```python
from build123d import *

# Parameters (mm, degrees)
SKETCH1_R           = 2
SKETCH1_R_2         = 1.5
BOSS_EXTRUDE1_DEPTH = 3.175


with BuildPart() as part:
    # Sketch1 → Boss-Extrude1 (new body)
    with BuildSketch(Plane.XY):
        with BuildLine():
            Line((165, 154), (165, 99))
            Line((165, 99), (151, 85))
            Line((151, 85), (151, -85))
            Line((151, -85), (165, -99))
            Line((165, -99), (165, -154))
            ThreePointArc((165, -154), (161.778174593, -161.778174593), (154, -165))
            Line((154, -165), (99, -165))
            Line((99, -165), (85, -151))
            Line((85, -151), (-85, -151))
            Line((-85, -151), (-99, -165))
            Line((-99, -165), (-154, -165))
            ThreePointArc((-154, -165), (-161.778174593, -161.778174593), (-165, -154))
            Line((-165, -154), (-165, -99))
            Line((-165, -99), (-151, -85))
            Line((-151, -85), (-151, 85))
            Line((-151, 85), (-165, 99))
            Line((-165, 99), (-165, 154))
            ThreePointArc((-165, 154), (-161.778174593, 161.778174593), (-154, 165))
            Line((-154, 165), (-64, 165))
            Line((-64, 165), (-60, 169))
            Line((-60, 169), (60, 169))
            Line((60, 169), (64, 165))
            Line((64, 165), (154, 165))
            ThreePointArc((154, 165), (161.778174593, 161.778174593), (165, 154))
        make_face()
        with Locations((-14.5, -0.5)):
            Circle(SKETCH1_R, mode=Mode.SUBTRACT)
        with Locations((-93, 64)):
            Circle(SKETCH1_R, mode=Mode.SUBTRACT)
        with Locations((-93, 39)):
            Circle(SKETCH1_R, mode=Mode.SUBTRACT)
        with Locations((-57, 39)):
            Circle(SKETCH1_R, mode=Mode.SUBTRACT)
        with Locations((-57, 64)):
            Circle(SKETCH1_R, mode=Mode.SUBTRACT)
        with Locations((57, 39)):
            Circle(SKETCH1_R, mode=Mode.SUBTRACT)
        with Locations((57, 64)):
            Circle(SKETCH1_R, mode=Mode.SUBTRACT)
        with Locations((93, 39)):
            Circle(SKETCH1_R, mode=Mode.SUBTRACT)
        with Locations((93, 64)):
            Circle(SKETCH1_R, mode=Mode.SUBTRACT)
        with Locations((57, -64)):
            Circle(SKETCH1_R, mode=Mode.SUBTRACT)
        with Locations((57, -39)):
            Circle(SKETCH1_R, mode=Mode.SUBTRACT)
        with Locations((93, -39)):
            Circle(SKETCH1_R, mode=Mode.SUBTRACT)
        with Locations((93, -64)):
            Circle(SKETCH1_R, mode=Mode.SUBTRACT)
        with Locations((-93, -64)):
            Circle(SKETCH1_R, mode=Mode.SUBTRACT)
        with Locations((-57, -64)):
            Circle(SKETCH1_R, mode=Mode.SUBTRACT)
        with Locations((-57, -39)):
            Circle(SKETCH1_R, mode=Mode.SUBTRACT)
        with Locations((-93, -39)):
            Circle(SKETCH1_R, mode=Mode.SUBTRACT)
        with Locations((-20.5, -26.5)):
            Circle(SKETCH1_R, mode=Mode.SUBTRACT)
        with Locations((-161.5, 154)):
            Circle(SKETCH1_R_2, mode=Mode.SUBTRACT)
        with Locations((-154, 161.5)):
            Circle(SKETCH1_R_2, mode=Mode.SUBTRACT)
        with Locations((154, 161.5)):
            Circle(SKETCH1_R_2, mode=Mode.SUBTRACT)
        with Locations((161.5, 154)):
            Circle(SKETCH1_R_2, mode=Mode.SUBTRACT)
        with Locations((161.5, -154)):
            Circle(SKETCH1_R_2, mode=Mode.SUBTRACT)
        with Locations((-20.5, 25.5)):
            Circle(SKETCH1_R, mode=Mode.SUBTRACT)
        with Locations((-25, -65.5)):
            Circle(SKETCH1_R, mode=Mode.SUBTRACT)
        with Locations((154, -161.5)):
            Circle(SKETCH1_R_2, mode=Mode.SUBTRACT)
        with Locations((-161.5, -154)):
            Circle(SKETCH1_R_2, mode=Mode.SUBTRACT)
        with Locations((-154, -161.5)):
            Circle(SKETCH1_R_2, mode=Mode.SUBTRACT)
        with Locations((-110, 95)):
            Circle(SKETCH1_R, mode=Mode.SUBTRACT)
        with Locations((-110, 83)):
            Circle(SKETCH1_R, mode=Mode.SUBTRACT)
        with Locations((-102, 89)):
            Circle(SKETCH1_R, mode=Mode.SUBTRACT)
        with Locations((-125, 83)):
            Circle(SKETCH1_R_2, mode=Mode.SUBTRACT)
        with Locations((-154, 154)):
            Circle(SKETCH1_R_2, mode=Mode.SUBTRACT)
        with Locations((154, 154)):
            Circle(SKETCH1_R_2, mode=Mode.SUBTRACT)
        with Locations((154, -154)):
            Circle(SKETCH1_R_2, mode=Mode.SUBTRACT)
        with Locations((-154, -154)):
            Circle(SKETCH1_R_2, mode=Mode.SUBTRACT)
        with Locations((-55, 161.5)):
            Circle(SKETCH1_R_2, mode=Mode.SUBTRACT)
        with Locations((55, 161.5)):
            Circle(SKETCH1_R_2, mode=Mode.SUBTRACT)
    extrude(amount=BOSS_EXTRUDE1_DEPTH)


solid = part.part
```
Model file for the job. Use its own axes, mm. A direction names the side the tool comes from. Coordinates: 2 decimals unless noted, no trailing zeros. Loops run counter-clockwise (first coordinate to the right, second up) from the corner with the lowest first, then second, coordinate; pieces in that order, holes last. Notation, with made-up numbers: (75.5, 7.25) -> (128.5, 7.25) arc R25 cw to (128.5, 20.25) -> close; hole circle Ø2 at (31.25, -26). An arc over 180 degrees is marked (long way). Answer as a JSON object with one key per item and string values.
Q1. 3-axis set-ups, long thin cutter, end or side, ignore diameter. For faces 4 (the flat face through (92, -158, 2)), 5 (the flat face through (158, -92, 2)), 6 (the flat face through (-158, 92, 2)), 7 (the flat face through (2, 4, 0)), 8 (the cylindrical face through (161.863, -161.692, 1.565)): which of +Z, -Z, +X, -X, +Y, -Y reach the whole face in a straight line?
Report:
{"face 4": "+Z, -Z, -Y", "face 5": "+Z, -Z, +X", "face 6": "+Z, -Z, -X", "face 7": "-Z, +X, -X, +Y, -Y", "face 8": "+Z, -Z, +X, -Y"}
Q2. Cut at A-A (z = 1). State how many separate pieces and enclosed holes the cut face has, and give its area (3 significant figures).
Report:
{"separate pieces": "1", "enclosed holes": "38", "area": "101,000 mm2"}
Q3. Cut at B-B (x = -75). List the corners of the cut face in (y, z) (3 decimals).
Report:
{"outline": "(-151, 0) -> (165, 0) -> (165, 3.175) -> (-151, 3.175) -> close"}
Q4. Pull direction Y, two halves, no side cores. Call faces 1 (the cylindrical face through (161.692, 161.863, 1.565)), 2 (the flat face through (-92, -158, 2)), 3 (the flat face through (-158, -92, 2)): released by +Y, released by -Y, zero draft, split by the parting line, or undercut.
Report:
{"face 1": "released by +Y", "face 2": "released by -Y", "face 3": "undercut"}
Q5. Probe probe 1 along Y at (x, z) = (-161.5, 1.6); probe 2 along Y at (x, z) = (-20.5, 1.25); probe 3 along Y at (x, z) = (-154, 0.8). List the from-to ranges inside material, lowest first.
Report:
{"probe 1": "y = -162.05 to -155.5, -152.5 to -95.5, 95.5 to 152.5, 155.5 to 162.05", "probe 2": "y = -151 to -28.5, -24.5 to 23.5, 27.5 to 169", "probe 3": "y = -165 to -163, -160 to -155.5, -152.5 to -88, 88 to 152.5, 155.5 to 160, 163 to 165"}
Q6. Flat gauge pins, fed straight in: P1, Ø5, axis at x = -102, y = 89, coming from the +Z side (3 decimals); P2, Ø1, axis at y = -40.5, z = 1, coming from the +X side. Where does each tip first touch, or does it go through?
Report:
{"P1": "stops at z = 3.175", "P2": "stops at x = 151"}
